from build123d import *

# Parameters (mm, degrees)
SKETCH_2_W          = 60
SKETCH_2_H          = 42
EXTRUDE_1_DEPTH     = 2.5
CUT_EXTRUDE_START   = 2.5
SKETCH_3_R          = 1.5
CUT_EXTRUDE_1_DEPTH = 2.5
SKETCH_6_W          = 40
SKETCH_6_H          = 10
CUT_EXTRUDE_2_DEPTH = 2.5
SKETCH_7_W          = 60
SKETCH_7_H          = 10
EXTRUDE_3_DEPTH     = 6
EXTRUDE_START       = 2.5
SKETCH_9_W          = 3
SKETCH_9_H          = 42
EXTRUDE_4_DEPTH     = 17.5
EXTRUDE_START_2     = 30
EXTRUDE_5_DEPTH     = 60
CUT_EXTRUDE_START_2 = 30
SKETCH_16_R         = 1.75
CUT_EXTRUDE_3_DEPTH = 3
CUT_EXTRUDE_START_3 = -30
CUT_EXTRUDE_4_DEPTH = 60
CHAMFER_1_SIZE      = 2
CUT_EXTRUDE_6_DEPTH = 63
CHAMFER_2_SIZE      = 2
CUT_EXTRUDE_START_4 = 33
SKETCH_21_W         = 20
SKETCH_21_H         = 10
CUT_EXTRUDE_7_DEPTH = 1
CHAMFER_3_SIZE      = 1
CHAMFER_4_SIZE      = 3


with BuildPart() as part:
    # 草图2 → 凸台-拉伸1 (new body)
    with BuildSketch(Plane(origin=(0, 0, 0), x_dir=(1, 0, 0), z_dir=(0, 1, 0))):
        Rectangle(SKETCH_2_W, SKETCH_2_H)
    extrude(amount=EXTRUDE_1_DEPTH)

    # 草图3 → 切除-拉伸1 (cut)
    with BuildSketch(Plane(origin=(0, 0, 0), x_dir=(1, 0, 0), z_dir=(0, 1, 0)).offset(CUT_EXTRUDE_START)):
        with Locations(Location((-25, 16, 0), (0, 0, 270))):
            Circle(SKETCH_3_R)
        with Locations(Location((25, 16, 0), (0, 0, 270))):
            Circle(SKETCH_3_R)
        with Locations(Location((-25, -16, 0), (0, 0, 270))):
            Circle(SKETCH_3_R)
        with Locations(Location((25, -16, 0), (0, 0, 270))):
            Circle(SKETCH_3_R)
    extrude(amount=-CUT_EXTRUDE_1_DEPTH, mode=Mode.SUBTRACT)

    # 草图6 → 切除-拉伸2 (cut)
    with BuildSketch(Plane(origin=(0, 0, 0), x_dir=(1, 0, 0), z_dir=(0, 1, 0))):
        with Locations((0, 16)):
            Rectangle(SKETCH_6_W, SKETCH_6_H)
        with Locations((0, -16)):
            Rectangle(SKETCH_6_W, SKETCH_6_H)
    extrude(amount=CUT_EXTRUDE_2_DEPTH, mode=Mode.SUBTRACT)

    # 草图7 → 凸台-拉伸3 (add)
    with BuildSketch(Plane(origin=(0, 0, 0), x_dir=(1, 0, 0), z_dir=(0, 1, 0))):
        Rectangle(SKETCH_7_W, SKETCH_7_H)
    extrude(amount=-EXTRUDE_3_DEPTH)

    # 草图9 → 凸台-拉伸4 (add)
    with BuildSketch(Plane(origin=(0, 0, 0), x_dir=(1, 0, 0), z_dir=(0, 1, 0)).offset(EXTRUDE_START)):
        with Locations((31.5, 0)):
            Rectangle(SKETCH_9_W, SKETCH_9_H)
    extrude(amount=-EXTRUDE_4_DEPTH)

    # 草图11 → 凸台-拉伸5 (add)
    with BuildSketch(Plane(origin=(0, 0, 0), x_dir=(0, 0, -1), z_dir=(1, 0, 0)).offset(EXTRUDE_START_2)):
        Polygon((5, -6), (11, 0), (5, 0), align=None)
        Polygon((-5, -6), (-5, 0), (-11, 0), align=None)
    extrude(amount=-EXTRUDE_5_DEPTH)

    # 草图16 → 切除-拉伸3 (cut)
    with BuildSketch(Plane(origin=(0, 0, 0), x_dir=(0, 0, -1), z_dir=(1, 0, 0)).offset(CUT_EXTRUDE_START_2)):
        with Locations(Location((-15.5, -11.5, 0), (0, 0, 180))):
            Circle(SKETCH_16_R)
        with Locations(Location((15.5, -11.5, 0), (0, 0, 180))):
            Circle(SKETCH_16_R)
    extrude(amount=CUT_EXTRUDE_3_DEPTH, mode=Mode.SUBTRACT)

    # 草图18 → 切除-拉伸4 (cut)
    with BuildSketch(Plane(origin=(0, 0, 0), x_dir=(0, 0, -1), z_dir=(1, 0, 0)).offset(CUT_EXTRUDE_START_3)):
        Polygon((6.171572875, -2), (4.171572875, -4), (-4.171572875, -4), (-6.171572875, -2), align=None)
    extrude(amount=CUT_EXTRUDE_4_DEPTH, mode=Mode.SUBTRACT)

    # 倒角1
    chamfer_1_edges = [part.edges().sort_by_distance(p)[0] for p in [
        (30, 0, -16),
        (30, -3, -8),
        (30, -3, 8),
        (30, 0, 16),
    ]]
    chamfer(chamfer_1_edges, length=CHAMFER_1_SIZE)

    # 草图19 → 切除-拉伸6 (cut)
    with BuildSketch(Plane(origin=(0, 0, 0), x_dir=(0, 0, -1), z_dir=(1, 0, 0)).offset(CUT_EXTRUDE_START_3)):
        Polygon((6.171572875, 2.5), (4.171572875, 0), (-4.171572875, 0), (-6.171572875, 2.5), align=None)
    extrude(amount=CUT_EXTRUDE_6_DEPTH, mode=Mode.SUBTRACT)

    # 倒角2
    chamfer_2_edges = [part.edges().sort_by_distance(p)[0] for p in [
        (20, 1.25, 21),
        (-20, 1.25, 21),
        (-20, 1.25, -21),
        (20, 1.25, -21),
        (-30, 1.25, 21),
        (-30, 1.25, -21),
        (31.5, -15, -21),
        (31.5, -15, 21),
    ]]
    chamfer(chamfer_2_edges, length=CHAMFER_2_SIZE)

    # 草图21 → 切除-拉伸7 (cut)
    with BuildSketch(Plane(origin=(0, 0, 0), x_dir=(0, 0, -1), z_dir=(1, 0, 0)).offset(CUT_EXTRUDE_START_4)):
        with Locations((0, -10)):
            Rectangle(SKETCH_21_W, SKETCH_21_H)
    extrude(amount=-CUT_EXTRUDE_7_DEPTH, mode=Mode.SUBTRACT)

    # 倒角3
    chamfer_3_edges = [part.edges().sort_by_distance(p)[0] for p in [
        (33, 2.5, 13.585786438),
        (33, 0, 0),
        (33, 1.25, -5.171572875),
        (33, 2.5, -13.585786438),
        (32, -10, -10),
        (32, -10, 10),
        (32, -5, 0),
    ]]
    chamfer(chamfer_3_edges, length=CHAMFER_3_SIZE - 0.0001)  # a hair under: the kernel refuses the full size

    # 倒角4
    chamfer_4_edges = [part.edges().sort_by_distance(p)[0] for p in [
        (-20, 1.25, 11),
        (20, 1.25, 11),
        (20, 1.25, -11),
        (-20, 1.25, -11),
    ]]
    chamfer(chamfer_4_edges, length=CHAMFER_4_SIZE)


solid = part.part
The model under review builds one solid part; all positions refer to its coordinate system, in mm. A direction names the side the tool comes from. Give positions to 0.01 mm unless a question says otherwise; leave off trailing zeros. Loops run counter-clockwise (first coordinate to the right, second up) from the corner with the lowest first, then second, coordinate; pieces in that order, holes last. Notation, with made-up numbers: (5.25, 34.25) -> (29.25, 34.25) arc R14 cw to (29.25, 43.25) -> close; hole circle Ø11 at (-26, 61). An arc over 180 degrees is marked (long way). Put each result on its own line as item: value. Start each with the question number.
1. We need section A-A on x = 25. State the section outline as (y, z) points, then the cut area to 3 significant figures.
2. Mouldability with a two-part tool opening along Y and no side actions: class faces 6 (the face through (0, 1, 11)), 7 (the face through (30, -3, 0)), 8 (the face through (31, -15, 0)) as released by +Y, released by -Y, zero draft, split by the parting line, or undercut.
3. For faces 1 (the face through (29, -1, -16)), 2 (the face through (-20, 1, 17)), 3 (the face through (1, 2.5, -10)), 4 (the face through (19, 1, -13)), 5 (the face through (32.507, 0.766, -5.433)), list the 3-axis set-ups (+Z, -Z, +X, -X, +Y, -Y) from which the entire face can be reached by the end or side of a thin tool; tool diameter is ignored.
4. Wall thickness on probe 1 along X at (y, z) = (1.25, -16); probe 2 along Z at (x, y) = (31.85, -11.5); probe 3 along Y at (x, z) = (-18, 2): over which ranges is each line inside the solid? List them lowest first.
5. We need section C-C on x = -4. State the section outline as (y, z) points, then the cut area to 3 significant figures.
6. We need section B-B on y = -11.5. State how many separate pieces and enclosed holes the cut face has, then the cut area to 3 significant figures.
7. We need section D-D on z = 16. State the section outline as (x, y) points.
8. Clearance check with flat-ended pins moving along their axes: P1, Ø0.6, axis at y = -3, z = -2, coming from the -X side; P2, Ø1.2, axis at x = -3.5, y = 1.5, coming from the -Z side; P3, Ø2, axis at y = -8.5, z = -2.5, coming from the +X side; P4, Ø2.5, axis at x = 25, z = 16, coming from the -Y side. State where each tip first meets the part, or that it passes through.
Determined:
1. outline: (-6, -5) -> (0, -11) -> (0, -14.5) -> (2.5, -14.5) -> (2.5, -6.17) -> (0, -4.17) -> (0, 4.17) -> (2.5, 6.17) -> (2.5, 14.5) -> (0, 14.5) -> (0, 11) -> (-6, 5) -> close; (0, -21) -> (2.5, -21) -> (2.5, -17.5) -> (0, -17.5) -> close; (0, 17.5) -> (2.5, 17.5) -> (2.5, 21) -> (0, 21) -> close; hole (-4, -4.17) -> (-2, -6.17) -> (-2, 6.17) -> (-4, 4.17) -> close
1. area: 139 mm^2
2. face 6: zero draft
2. face 7: undercut
2. face 8: released by -Y
3. face 1: -Z, -X, -Y
3. face 2: +Z, +Y, -Y
3. face 3: +Z, -Z, +X, -X, +Y
3. face 4: -Z, +Y, -Y
3. face 5: +X, +Y
4. probe 1: -30 to -26.5, -23.5 to -20, 20 to 23.5, 26.5 to 33
4. probe 2: -21 to -17.25, -13.75 to 13.75, 17.25 to 21
4. probe 3: -6 to -4, -2 to 0
5. outline: (-6, -5) -> (0, -11) -> (2.5, -11) -> (2.5, -6.17) -> (0, -4.17) -> (0, 4.17) -> (2.5, 6.17) -> (2.5, 11) -> (0, 11) -> (-6, 5) -> close; hole (-4, -4.17) -> (-2, -6.17) -> (-2, 6.17) -> (-4, 4.17) -> close
5. area: 104 mm^2
6. separate pieces: 3
6. enclosed holes: 0
6. area: 86.0 mm^2
7. outline: (-30, 0) -> (-26.5, 0) -> (-26.5, 2.5) -> (-30, 2.5) -> close; (-23.5, 0) -> (-20, 0) -> (-20, 2.5) -> (-23.5, 2.5) -> close; (20, 0) -> (23.5, 0) -> (23.5, 2.5) -> (20, 2.5) -> close; (26.5, 0) -> (28, 0) -> (30, -2) -> (30, -9.82) -> (33, -9.82) -> (33, 1.5) -> (32, 2.5) -> (26.5, 2.5) -> close; (30, -15) -> (33, -15) -> (33, -13.18) -> (30, -13.18) -> close
8. P1: x = 30
8. P2: z = -11
8. P3: x = 32
8. P4: through
